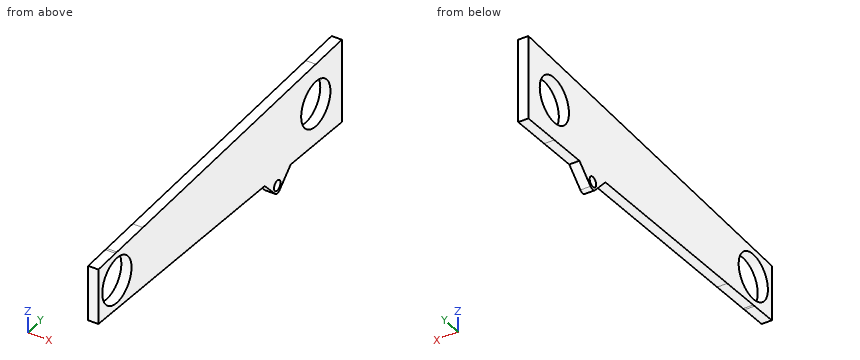
Autodesk Inventor part; units mm, degrees
ref_plane "YZ Plane" through (0, 0, 0) normal (1, 0, 0) x (0, 1, 0)
ref_plane "XZ Plane" through (0, 0, 0) normal (0, 1, 0) x (-1, 0, 0)
ref_plane "XY Plane" through (0, 0, 0) normal (0, 0, 1) x (1, 0, 0)
sketch "Sketch1" plane through (0, 0, 0) normal (1, 0, 0) x (0, 1, 0)
  line L0 (0, -38.1) -> (169.0878, -44.45)
  line L1 (169.0878, -44.45) -> (169.0878, 6.35)
  line L2 (169.0878, 6.35) -> (0, 0)
  line L3 (0, 0) -> (0, -38.1)
  arc A0 (169.0878, -44.45) -> (169.0878, 6.35) centre (169.0878, -19.05) ccw
  circle A1 centre (169.0878, -19.05) radius 14.2875
  point P0 (0, -19.05)
  point P1 (169.0878, -33.3375)
  point P2 (169.0878, -4.7625)
  dimension "d3" = 50.8
  dimension "d4" = 38.1
  dimension "d5" = 28.575
  dimension "d9" = 169.0878
extrude "Extrusion1" add sketch "Sketch1" against normal blind 6.35 contours L3 L2 L1 A1 L0 | L1 A1 A0
sketch "Sketch3" plane through (-6.35, 0, 0) normal (-1, 0, 0) x (0, 0, 1)
  line L0 (-38.1, 0) -> (0, 0)
  line L1 (0, 0) -> (-0.9539, -25.4)
  line L2 (-44.45, 169.0878) -> (-38.1, 0)
  line L3 (-38.1, 0) -> (-37.1461, -25.4)
  line L4 (0, 0) -> (6.35, 169.0878)
  line L5 (-37.1461, -25.4) -> (-0.9539, -25.4)
  arc A0 (-37.1461, -25.4) -> (-0.9539, -25.4) centre (-19.05, -25.4) ccw
  circle A1 centre (-19.05, -25.4) radius 14.2875
  dimension "d12" = 25.4
  dimension "d13" = 28.575
extrude "Extrusion2" add sketch "Sketch3" against normal blind 6.35 contours L0 L1 L5 A1 L3 | L5 A1 A0
sketch "Sketch4" plane through (-6.35, 0, 0) normal (-1, 0, 0) x (0, 0, 1)
  line L0 (6.35, 169.0878) -> (-0.9539, -25.4)
  line L1 (-0.9539, -25.4) -> (-1.6335, -43.4961)
  line L2 (-37.1461, -25.4) -> (-44.45, 169.0878)
  line L3 (-37.1461, -25.4) -> (-36.4665, -43.4961)
  arc A0 (-37.1461, -25.4) -> (-0.9539, -25.4) centre (-19.05, -25.4) ccw
  line L4 (-1.6335, -43.4961) -> (-36.4665, -43.4961)
  line L5 (6.35, 169.0878) -> (7.3039, 194.4878)
  line L6 (-44.45, 169.0878) -> (-45.4039, 194.4878)
  arc A1 (6.35, 169.0878) -> (-44.45, 169.0878) centre (-19.05, 169.0878) ccw
  line L7 (7.3039, 194.4878) -> (-45.4039, 194.4878)
  point P0 (0, 0)
  point P1 (-19.05, -43.4961)
  point P2 (-19.05, -43.4961)
  point P3 (-19.05, 194.4878)
  point P4 (-19.05, 194.4878)
  point P5 (-19.05, -43.4961)
  point P6 (-1.0049, -26.7573)
  point P7 (-37.0951, -26.7573)
  point P8 (-19.05, 194.4878)
extrude "Extrusion3" add sketch "Sketch4" against normal blind 6.35 contours A1 L7 L5 | A1 L6 L7 | L1 L4 A0 | L4 L3 A0
sketch "Sketch5" plane through (-6.35, 0, 0) normal (-1, 0, 0) x (0, 0, 1)
  circle A0 centre (-49.393, 131.3829) radius 3.175
  line L0 (-36.4665, -43.4961) -> (-1.6335, -43.4961)
  line L1 (-0.9539, -25.4) -> (7.3039, 194.4878)
  line L2 (-45.4039, 194.4878) -> (-37.1461, -25.4)
  line L3 (-43.5289, 144.5595) -> (-55.743, 131.3829)
  line L4 (-55.743, 131.3829) -> (-42.575, 119.1595)
  point P0 (0, 0)
  dimension "d18" = 6.35
  dimension "d19" = 174.879
  dimension "d29" = 25.4
  dimension "d30" = 12.7
  dimension "d31" = 6.35
extrude "Extrusion4" add sketch "Sketch5" against normal blind 6.35
fillet "Fillet1" radius 3.175 1 edges at (-3.175, 131.3829, -55.743)
properties part number "Intake - Side Panel"
Geometry: final body of the model. Coordinates: model frame, mm. Give positions to 0.01 mm unless a question says otherwise; leave off trailing zeros. Write each loop counter-clockwise with the first axis right and the second up, starting at its lowest first coordinate (ties: lowest second). Pieces come first, ordered by that corner, then holes.
1. Pin query (flat end, axial travel): P1, Ø1, axis at x = -3, y = 95, coming from the -Z side. Return the tip coordinate at first contact, or that it passes through.
2. Section query D-D, the plane y = 150.5. Return loops of the section in (x, z).
3. Section query C-C, the plane y = 53. Return loops of the section in (x, z), then the cut area to 3 significant figures.
4. Line query: probe 1 along Y at (x, z) = (-1.5, -19.05); probe 2 along Z at (x, y) = (-4.5, -25.4); probe 3 along Y at (x, z) = (-1.25, -16.5). Output: solid intervals per line, ascending.
5. Section query B-B, the plane x = -1.25. Count the separate pieces of the cut face and the enclosed holes in it, then the cut area to 3 significant figures.
6. Section query A-A, the plane z = -19.05. Return loops of the section in (x, y), then the cut area to 3 significant figures.
Computed:
1. P1: stops at z = -41.69
2. outline: (-6.35, -43.75) - (0, -43.75) - (0, 5.65) - (-6.35, 5.65) - close
3. outline: (-6.35, -40.09) - (0, -40.09) - (0, 1.99) - (-6.35, 1.99) - close
3. area: 267 mm2
4. probe 1: y = -43.5 to -39.69, -11.11 to 154.8, 183.38 to 194.49
4. probe 2: z = -37.15 to -33.34, -4.76 to -0.95
4. probe 3: y = -43.5 to -39.46, -11.34 to 155.03, 183.15 to 194.49
5. separate pieces: 1
5. enclosed holes: 3
5. area: 9,260 mm2
6. outline: (-6.35, -43.5) - (0, -43.5) - (0, -39.69) - (-6.35, -39.69) - close; (-6.35, -11.11) - (0, -11.11) - (0, 154.8) - (-6.35, 154.8) - close; (-6.35, 183.38) - (0, 183.38) - (0, 194.49) - (-6.35, 194.49) - close
6. area: 1,150 mm2
